```python
from build123d import *

# Parameters (mm, degrees)
F0_W     = 40
F0_H     = 25
F1_DEPTH = 49.3
F2_R     = 19.99999
F3_SIZE  = 5


# Not quite as in the source:
# - a fillet or chamfer is up to 0.001 mm smaller than in the source, because OpenCascade refuses the exact size


with BuildPart() as f1:
    # F0 (on Top) → F1 (new body)
    with BuildSketch(Plane.XY):
        with Locations((-24.3057886145, -13.9031428844)):
            Rectangle(F0_W, F0_H)
    extrude(amount=F1_DEPTH)

    # F2 (radius 20 in the source; OpenCascade refuses exactly that, so slightly less here)
    f2_edges = [f1.edges().sort_by_distance(p)[0] for p in [
        (-44.305789, -26.403143, 24.65),
        (-4.305789, -26.403143, 24.65),
        (-24.305789, -26.403143, 0),
        (-24.305789, -26.403143, 49.3),
    ]]
    fillet(f2_edges, radius=F2_R)

    # F3
    f3_edges = [f1.edges().sort_by_distance(p)[0] for p in [
        (-4.305789, -1.403143, 24.65),
        (-44.305789, -1.403143, 24.65),
        (-24.305789, -1.403143, 0),
        (-24.305789, -1.403143, 49.3),
    ]]
    chamfer(f3_edges, length=F3_SIZE)


solid = f1.part
```
Input: part model. Units: mm. Frame: model coordinates. Give positions to 0.01 mm unless a question says otherwise; leave off trailing zeros. Order: outer loops, then holes, each group sorted by start corner. A loop starts at its lowest first (then second) coordinate and runs counter-clockwise, first axis right, second up. Notation, with made-up numbers: M -7,49 L 9,49 A7 cw 9,57 Z; hole C 30,26 d5. An arc over 180 degrees is marked long. One line per question, with ' | ' between items. Start each with the question number.
1. Section query D-D (y = -23). Return the cut outline in (x, z).
2. Material intervals for probe 1 along Y at (x, z) = (-35.5, 30); probe 2 along Z at (x, y) = (-23, -20.75); probe 3 along Y at (x, z) = (-18, 21), sorted ascending. Write a range as [from, to].
3. Section query C-C (y = -5.75). Return the cut outline in (x, z).
4. First-contact query: pin 1 Ø2 at (x, y) = (-24, -13) entering from +Z; pin 2 Ø6 at (x, y) = (-39.5, -14) entering from +Z; pin 3 Ø2 at (y, z) = (-17, 40) entering from +X. Flat tips, straight axial feed; report the tip coordinate or a pass-through.
5. Pull-direction query (Y, two-part tool) for faces 1 (the face through (-25, -1.403, 24)), 2 (the face through (-24.03, -18.05, 3.74)); classes: released by +Y, released by -Y, zero draft, split by the parting line, or undercut.
Here are the results:
1) outline: M -35.47,8.84 L -13.15,8.84 L -13.15,40.46 L -35.47,40.46 Z
2) probe 1: [-22.98, -1.4] | probe 2: [6.07, 43.23] | probe 3: [-25.38, -1.4]
3) outline: M -43.65,0.65 L -4.96,0.65 L -4.96,48.65 L -43.65,48.65 Z
4) pin 1: z = 48.5 | pin 2: z = 48.76 | pin 3: x = -6.76
5) face 1: released by +Y | face 2: released by -Y
